from build123d import *

# Parameters (mm, degrees)
EXTRUDE_1_DEPTH = 42.75


with BuildPart() as part:
    # ｽｹｯﾁ1 → ﾎﾞｽ - 押し出し1 (new, symmetric)
    with BuildSketch(Plane.XY):
        with BuildLine():
            Line((33, 0), (-33, 0))
            ThreePointArc((-33, 0), (-36.75647589, -2.625631458), (-35.581391146, -7.055555556))
            ThreePointArc((-35.581391146, -7.055555556), (-34.748138628, -7.207150732), (-34.197540305, -6.563619582))
            ThreePointArc((-34.197540305, -6.563619582), (-34.230384711, -6.483196795), (-34.317201966, -6.480140047))
            ThreePointArc((-34.317201966, -6.480140047), (-34.687300356, -6.562097055), (-35.032845527, -6.40625))
            ThreePointArc((-35.032845527, -6.40625), (-35.794525899, -3.108842358), (-33, -1.2))
            Line((-33, -1.2), (33, -1.2))
            ThreePointArc((33, -1.2), (35.794525899, -3.108842358), (35.032845527, -6.40625))
            ThreePointArc((35.032845527, -6.40625), (34.687300356, -6.562097055), (34.317201966, -6.480140047))
            ThreePointArc((34.317201966, -6.480140047), (34.230384711, -6.483196795), (34.197540305, -6.563619582))
            ThreePointArc((34.197540305, -6.563619582), (34.748138628, -7.207150732), (35.581391146, -7.055555556))
            ThreePointArc((35.581391146, -7.055555556), (36.75647589, -2.625631458), (33, 0))
        make_face()
    extrude(amount=EXTRUDE_1_DEPTH, both=True)


solid = part.part
Can you work these out from the model? Positions are in its coordinate system, mm. A direction names the side the tool comes from. Round coordinates to 2 decimals unless told otherwise and drop trailing zeros. Write each loop counter-clockwise with the first axis right and the second up, starting at its lowest first coordinate (ties: lowest second). Pieces come first, ordered by that corner, then holes. Notation, with made-up numbers: (69.25, -10) - (73.25, -10) arc R28 cw to (73.25, 23) - close; hole circle Ø2 at (67.5, 56.5). An arc over 180 degrees is marked (long way). Write each question's results on one line, items separated by ' | '. Start each with the question number.
1) Suppose I cut it at C-C (z = -18). List the corners of the cut face in (x, y) for me.
2) We'd pull the mould along X, two halves only. Please class faces 4 (the flat face through (0, 0, 1)), 5 (the cylindrical face through (-35.812, -3.156, 0.599)), 6 (the cylindrical face through (36.78, -2.69, 0.6)): released by +X, released by -X, zero draft, split by the parting line, or undercut.
3) Please list where these lines run through material, in increasing order: line 1 (Y direction, x = 17.5, z = -26.5); line 2 (X direction, y = -2.75, z = 2); line 3 (X direction, y = -4.75, z = -8).
4) For pin 1 Ø6 at (x, z) = (-7.5, 27.5) entering from -Y; pin 2 Ø1 at (y, z) = (-5.5, -11.5) entering from +X, each with a flat end and sliding along its axis, tell me the tip position at first contact or that it passes through.
5) Suppose I cut it at A-A (y = -2.75). List the corners of the cut face in (x, z) for me.
6) Which directions (+Z, -Z, +X, -X, +Y, -Y) give clear straight access to the entire face, cutting with the end or side of a thin tool? Please do faces 1 (the flat face through (0, -1.2, 1)), 2 (the cylindrical face through (-36.73, -2.56, 0.6)), 3 (the cylindrical face through (35.776, -3.062, 0.599)).
7) Suppose I cut it at B-B (x = 19.5). List the corners of the cut face in (y, z) for me, and give its area (3 significant figures).
Here are the results:
1) outline: (-35.58, -7.06) arc R0.85 ccw to (-34.2, -6.56) arc R0.08 ccw to (-34.32, -6.48) arc R0.6 cw to (-35.03, -6.41) arc R3 cw to (-33, -1.2) - (33, -1.2) arc R3 cw to (35.03, -6.41) arc R0.6 cw to (34.32, -6.48) arc R0.08 ccw to (34.2, -6.56) arc R0.85 ccw to (35.58, -7.06) arc R4 ccw to (33, 0) - (-33, 0) arc R4 ccw to start
2) face 4: zero draft | face 5: undercut | face 6: released by +X
3) line 1: y = -1.2 to 0 | line 2: x = -36.8 to -35.63, 35.63 to 36.8 | line 3: x = -36.93 to -35.95, 35.95 to 36.93
4) pin 1: stops at y = -1.2 | pin 2: stops at x = 36.87
5) outline: (-36.8, -42.75) - (-35.63, -42.75) - (-35.63, 42.75) - (-36.8, 42.75) - close; (35.63, -42.75) - (36.8, -42.75) - (36.8, 42.75) - (35.63, 42.75) - close
6) face 1: +Z, -Z, -Y | face 2: +Z, -Z, -X | face 3: +Z, -Z
7) outline: (-1.2, -42.75) - (0, -42.75) - (0, 42.75) - (-1.2, 42.75) - close | area: 103 mm2
